Input: part model. Units: mm. Frame: model coordinates. Face numbers are marked on the shaded views. A direction names the side the tool comes from. Coordinates: 2 decimals unless noted, no trailing zeros. Order: outer loops, then holes, each group sorted by start corner. A loop starts at its lowest first (then second) coordinate and runs counter-clockwise, first axis right, second up. Notation, with made-up numbers: (87.5, 22) -> (125.5, 22) arc R22 ccw to (125.5, 51) -> close; hole circle Ø2 at (-6, -23). An arc over 180 degrees is marked (long way). Use one line per item in the form item = value. Start each with the question number.
1) Section query C-C on z = 0.5. Output: boundary loops of the cut face in (x, y).
2) Ray query, line 1 along Y through (x, z) = (-2.5, 0.5); line 2 along X through (y, z) = (14, -8); line 3 along Y through (x, z) = (0.25, 7.25). Return the intervals inside material, ascending.
3) Access query for the marked faces 1 and 2. Directions: +Z, -Z, +X, -X, +Y, -Y. A direction counts if a zero-diameter tool reaches every point of the face in a straight line with its end or side. Return the directions, or none.
4) Draft query along X for the marked faces 3, 4 and 5. Return one class per face: pulls with the +X half, pulls with the -X half, needs draft (parallel to the pull), parting line crosses it, or undercut.
5) Section query D-D on y = 1.75. Output: boundary loops of the cut face in (x, z), then the cut area to 3 significant figures.
6) Pin query (flat end, axial travel): pin 1 (0.8 mm diameter, centred on x = 0, z = 0, fed in from -Y); pin 2 (1 mm diameter, centred on x = 6, y = 10, fed in from +Z); pin 3 (1.5 mm diameter, centred on x = -2.5, y = 3.5, fed in from -Z). Return the tip coordinate at first contact, or that it passes through.
7) Section query B-B on y = 5.25. Output: boundary loops of the cut face in (x, z).
8) Section query A-A on x = 0. Output: boundary loops of the cut face in (y, z), then the cut area to 3 significant figures.
from build123d import *

# Parameters (mm, degrees)
SKETCH_1_R          = 2.5
EXTRUDE_1_DEPTH     = 6
SKETCH_2_R          = 3
EXTRUDE_2_DEPTH     = 1
SKETCH_3_R          = 2.5
EXTRUDE_3_DEPTH     = 2.5
SKETCH_4_R          = 8
EXTRUDE_4_DEPTH     = 8
SKETCH_6_R          = 0.5
EXTRUDE_5_DEPTH     = 8
SKETCH_7_R          = 0.5
CUT_EXTRUDE_1_DEPTH = 8
CUT_EXTRUDE_2_DEPTH = 1.5


with BuildPart() as part:
    # 草图1 → 凸台-拉伸1 (new body)
    with BuildSketch(Plane(origin=(0, 0, 0), x_dir=(1, 0, 0), z_dir=(0, 1, 0))):
        with Locations(Location((0, 0, 0), (0, 0, 270))):
            Circle(SKETCH_1_R)
    extrude(amount=EXTRUDE_1_DEPTH)

    # 草图2 → 凸台-拉伸2 (add)
    with BuildSketch(Plane(origin=(0, 6, 0), x_dir=(1, 0, 0), z_dir=(0, 1, 0))):
        with Locations(Location((0, 0, 0), (0, 0, 270))):
            Circle(SKETCH_2_R)
    extrude(amount=-EXTRUDE_2_DEPTH)

    # 草图3 → 凸台-拉伸3 (add)
    with BuildSketch(Plane(origin=(0, 6, 0), x_dir=(1, 0, 0), z_dir=(0, 1, 0))):
        with Locations(Location((0, 0, 0), (0, 0, 270))):
            Circle(SKETCH_3_R)
    extrude(amount=EXTRUDE_3_DEPTH)

    # 草图4 → 凸台-拉伸4 (add)
    with BuildSketch(Plane(origin=(0, 8.5, 0), x_dir=(1, 0, 0), z_dir=(0, 1, 0))):
        with Locations(Location((0, 0, 0), (0, 0, 270))):
            Circle(SKETCH_4_R)
    extrude(amount=EXTRUDE_4_DEPTH)

    # 草图6 → 凸台-拉伸5 (add)
    with BuildSketch(Plane(origin=(0, 16.5, 0), x_dir=(1, 0, 0), z_dir=(0, 1, 0))):
        with Locations((0, 8)):
            Circle(SKETCH_6_R)
        with Locations((1.989519097, 7.748665289)):
            Circle(SKETCH_6_R)
        with Locations((3.854029393, 7.01045344)):
            Circle(SKETCH_6_R)
        with Locations((5.476376847, 5.831749019)):
            Circle(SKETCH_6_R)
        with Locations((6.754623404, 4.28661436)):
            Circle(SKETCH_6_R)
        with Locations((7.60845213, 2.472135955)):
            Circle(SKETCH_6_R)
        with Locations((7.984213827, 0.502324156)):
            Circle(SKETCH_6_R)
        with Locations((7.858298006, -1.499050517)):
            Circle(SKETCH_6_R)
        with Locations((7.23861642, -3.406234333)):
            Circle(SKETCH_6_R)
        with Locations((6.164105942, -5.099391918)):
            Circle(SKETCH_6_R)
        with Locations((4.702282018, -6.472135955)):
            Circle(SKETCH_6_R)
        with Locations((2.944996421, -7.438211887)):
            Circle(SKETCH_6_R)
        with Locations((1.002665869, -7.936917611)):
            Circle(SKETCH_6_R)
        with Locations((-1.002665869, -7.936917611)):
            Circle(SKETCH_6_R)
        with Locations((-2.944996421, -7.438211887)):
            Circle(SKETCH_6_R)
        with Locations((-4.702282018, -6.472135955)):
            Circle(SKETCH_6_R)
        with Locations((-6.164105942, -5.099391918)):
            Circle(SKETCH_6_R)
        with Locations((-7.23861642, -3.406234333)):
            Circle(SKETCH_6_R)
        with Locations((-7.858298006, -1.499050517)):
            Circle(SKETCH_6_R)
        with Locations((-7.984213827, 0.502324156)):
            Circle(SKETCH_6_R)
        with Locations((-7.60845213, 2.472135955)):
            Circle(SKETCH_6_R)
        with Locations((-6.754623404, 4.28661436)):
            Circle(SKETCH_6_R)
        with Locations((-5.476376847, 5.831749019)):
            Circle(SKETCH_6_R)
        with Locations((-3.854029393, 7.01045344)):
            Circle(SKETCH_6_R)
        with Locations((-1.989519097, 7.748665289)):
            Circle(SKETCH_6_R)
    extrude(amount=-EXTRUDE_5_DEPTH)

    # 草图7 → 切除-拉伸1 (cut)
    with BuildSketch(Plane(origin=(0, 16.5, 0), x_dir=(1, 0, 0), z_dir=(0, 1, 0))):
        with Locations((1.002665869, 7.936917611)):
            Circle(SKETCH_7_R)
        with Locations((2.944996421, 7.438211887)):
            Circle(SKETCH_7_R)
        with Locations((4.702282018, 6.472135955)):
            Circle(SKETCH_7_R)
        with Locations((6.164105942, 5.099391918)):
            Circle(SKETCH_7_R)
        with Locations((7.23861642, 3.406234333)):
            Circle(SKETCH_7_R)
        with Locations((7.858298006, 1.499050517)):
            Circle(SKETCH_7_R)
        with Locations((7.984213827, -0.502324156)):
            Circle(SKETCH_7_R)
        with Locations((7.60845213, -2.472135955)):
            Circle(SKETCH_7_R)
        with Locations((6.754623404, -4.28661436)):
            Circle(SKETCH_7_R)
        with Locations((5.476376847, -5.831749019)):
            Circle(SKETCH_7_R)
        with Locations((3.854029393, -7.01045344)):
            Circle(SKETCH_7_R)
        with Locations((1.989519097, -7.748665289)):
            Circle(SKETCH_7_R)
        with Locations((0, -8)):
            Circle(SKETCH_7_R)
        with Locations((-1.989519097, -7.748665289)):
            Circle(SKETCH_7_R)
        with Locations((-3.854029393, -7.01045344)):
            Circle(SKETCH_7_R)
        with Locations((-5.476376847, -5.831749019)):
            Circle(SKETCH_7_R)
        with Locations((-6.754623404, -4.28661436)):
            Circle(SKETCH_7_R)
        with Locations((-7.60845213, -2.472135955)):
            Circle(SKETCH_7_R)
        with Locations((-7.984213827, -0.502324156)):
            Circle(SKETCH_7_R)
        with Locations((-7.858298006, 1.499050517)):
            Circle(SKETCH_7_R)
        with Locations((-7.23861642, 3.406234333)):
            Circle(SKETCH_7_R)
        with Locations((-6.164105942, 5.099391918)):
            Circle(SKETCH_7_R)
        with Locations((-4.702282018, 6.472135955)):
            Circle(SKETCH_7_R)
        with Locations((-2.944996421, 7.438211887)):
            Circle(SKETCH_7_R)
        with Locations((-1.002665869, 7.936917611)):
            Circle(SKETCH_7_R)
    extrude(amount=-CUT_EXTRUDE_1_DEPTH, mode=Mode.SUBTRACT)

    # 草图9 → 切除-拉伸2 (cut)
    with BuildSketch(Plane.XZ):
        with BuildLine():
            Line((-0.844097151, 1.3), (0.844097151, 1.3))
            ThreePointArc((0.844097151, 1.3), (1.55, 0), (0.844097151, -1.3))
            Line((0.844097151, -1.3), (-0.844097151, -1.3))
            ThreePointArc((-0.844097151, -1.3), (-1.55, 0), (-0.844097151, 1.3))
        make_face()
    extrude(amount=-CUT_EXTRUDE_2_DEPTH, mode=Mode.SUBTRACT)


solid = part.part
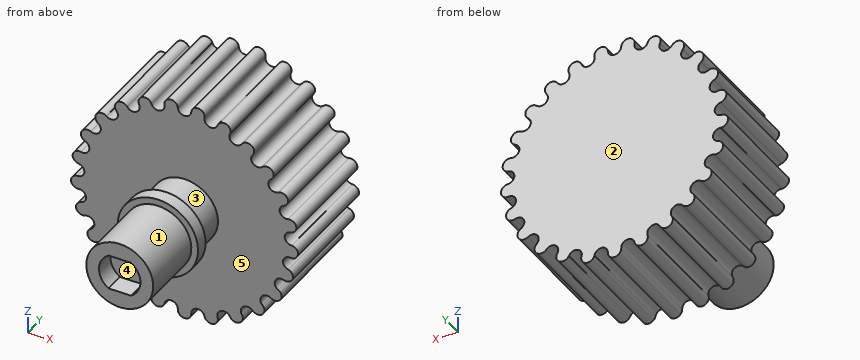
Answers below:
q1.outline = (-7.48, 8.5) -> (-2.45, 8.5) -> (-2.45, 6) -> (-2.96, 6) -> (-2.96, 5) -> (-2.45, 5) -> (-2.45, 0) -> (-1.47, 0) -> (-1.47, 1.5) -> (1.47, 1.5) -> (1.47, 0) -> (2.45, 0) -> (2.45, 5) -> (2.96, 5) -> (2.96, 6) -> (2.45, 6) -> (2.45, 8.5) -> (7.48, 8.5) -> (7.48, 16.5) -> (-7.48, 16.5) -> close
q2.line_1 = 5 to 6, 8.5 to 16.5
q2.line_2 = -2.42 to -1.56, -0.5 to 0.5, 1.56 to 2.42
q2.line_3 = 8.5 to 16.5
q3.face_1 = -Y
q3.face_2 = +Z, -Z, +X, -X, +Y
q4.face_3 = parting line crosses it
q4.face_4 = undercut
q4.face_5 = needs draft
q5.outline = circle Ø5 at (0, 0)
q5.area = 19.6 mm^2
q6.pin_1 = 1.5
q6.pin_2 = 5.6
q6.pin_3 = -1.79
q7.outline = circle Ø6 at (0, 0)
q8.outline = (0, -2.5) -> (5, -2.5) -> (5, -3) -> (6, -3) -> (6, -2.5) -> (8.5, -2.5) -> (8.5, -8.5) -> (16.5, -8.5) -> (16.5, 7.5) -> (8.5, 7.5) -> (8.5, 2.5) -> (6, 2.5) -> (6, 3) -> (5, 3) -> (5, 2.5) -> (0, 2.5) -> (0, 1.3) -> (1.5, 1.3) -> (1.5, -1.3) -> (0, -1.3) -> close
q8.area = 168 mm^2
